CAD build for the part. Positions are in the model's coordinates, mm. A direction names the side the tool comes from. Coordinates: 2 decimals unless noted, no trailing zeros. Loops run counter-clockwise (first coordinate to the right, second up) from the corner with the lowest first, then second, coordinate; pieces in that order, holes last. Notation, with made-up numbers: (-35.5, 48) -> (-21.5, 48) arc R17 cw to (-21.5, 79) -> close; hole circle Ø8 at (-20.75, 21). An arc over 180 degrees is marked (long way). Write each question's results on one line, items separated by ' | '.
```python
from build123d import *

# Parameters (mm, degrees)
SKETCH1_W           = 51.2
SKETCH1_H           = 37.6
BOSS_EXTRUDE1_DEPTH = 2
SKETCH2_W           = 2
SKETCH2_H           = 37.6
BOSS_EXTRUDE2_DEPTH = 37.6
SKETCH3_R           = 1.65
CUT_EXTRUDE2_DEPTH  = 37.6
SKETCH5_R           = 6.6
CUT_EXTRUDE3_DEPTH  = 37.6
SKETCH6_R           = 1.6
CUT_EXTRUDE4_DEPTH  = 37.6
FILLET1_R           = 2
FILLET2_R           = 2
FILLET3_R           = 18.8


with BuildPart() as part:
    # Sketch1 → Boss-Extrude1 (new body)
    with BuildSketch(Plane(origin=(0, 0, 0), x_dir=(1, 0, 0), z_dir=(0, 1, 0))):
        Rectangle(SKETCH1_W, SKETCH1_H)
    extrude(amount=BOSS_EXTRUDE1_DEPTH)

    # Sketch2 → Boss-Extrude2 (add)
    with BuildSketch(Plane(origin=(0, 2, 0), x_dir=(1, 0, 0), z_dir=(0, 1, 0))):
        with Locations((-24.6, 0)):
            Rectangle(SKETCH2_W, SKETCH2_H)
    extrude(amount=BOSS_EXTRUDE2_DEPTH)

    # Sketch3 → Cut-Extrude2 (cut)
    with BuildSketch(Plane.ZY.offset(25.6)):
        with Locations((15.5, 20.8)):
            Circle(SKETCH3_R)
        with Locations((6.883974596, 7.876606241)):
            Circle(SKETCH3_R)
        with Locations((-8.616025404, 8.876606241)):
            Circle(SKETCH3_R)
        with Locations((-15.5, 22.8)):
            Circle(SKETCH3_R)
        with Locations((-6.883974596, 35.723393759)):
            Circle(SKETCH3_R)
        with Locations((8.616025404, 34.723393759)):
            Circle(SKETCH3_R)
    extrude(amount=-CUT_EXTRUDE2_DEPTH, mode=Mode.SUBTRACT)

    # Sketch5 → Cut-Extrude3 (cut)
    with BuildSketch(Plane.ZY.offset(25.6)):
        with Locations((0, 27.8)):
            Circle(SKETCH5_R)
        with BuildLine():
            Line((6.6, 13.8), (6.6, 27.8))
            ThreePointArc((6.6, 27.8), (0, 21.2), (-6.6, 27.8))
            Line((-6.6, 27.8), (-6.6, 13.8))
            ThreePointArc((-6.6, 13.8), (0, 20.4), (6.6, 13.8))
        make_face()
        with Locations((0, 13.8)):
            Circle(SKETCH5_R)
    extrude(amount=-CUT_EXTRUDE3_DEPTH, mode=Mode.SUBTRACT)

    # Sketch6 → Cut-Extrude4 (cut)
    with BuildSketch(Plane(origin=(0, 0, 0), x_dir=(-1, 0, 0), z_dir=(0, -1, 0))):
        with Locations(Location((17.2, -15.6, 0), (0, 0, 90))):
            Circle(SKETCH6_R)
        with Locations(Location((10.8, -15.6, 0), (0, 0, 90))):
            Circle(SKETCH6_R)
        with Locations(Location((4.4, -15.6, 0), (0, 0, 90))):
            Circle(SKETCH6_R)
        with Locations(Location((-2, -15.6, 0), (0, 0, 90))):
            Circle(SKETCH6_R)
        with Locations(Location((-8.4, -15.6, 0), (0, 0, 90))):
            Circle(SKETCH6_R)
        with Locations(Location((-14.8, -15.6, 0), (0, 0, 90))):
            Circle(SKETCH6_R)
        with Locations(Location((-21.2, -15.6, 0), (0, 0, 90))):
            Circle(SKETCH6_R)
        with Locations(Location((-21.2, 15.6, 0), (0, 0, 270))):
            Circle(SKETCH6_R)
        with Locations(Location((-14.8, 15.6, 0), (0, 0, 270))):
            Circle(SKETCH6_R)
        with Locations(Location((-8.4, 15.6, 0), (0, 0, 270))):
            Circle(SKETCH6_R)
        with Locations(Location((-2, 15.6, 0), (0, 0, 270))):
            Circle(SKETCH6_R)
        with Locations(Location((4.4, 15.6, 0), (0, 0, 270))):
            Circle(SKETCH6_R)
        with Locations(Location((10.8, 15.6, 0), (0, 0, 270))):
            Circle(SKETCH6_R)
        with Locations(Location((17.2, 15.6, 0), (0, 0, 270))):
            Circle(SKETCH6_R)
    extrude(amount=-CUT_EXTRUDE4_DEPTH, mode=Mode.SUBTRACT)

    # Fillet1
    fillet1_edges = [part.edges().sort_by_distance(p)[0] for p in [
        (25.6, 1, -18.8),
        (25.6, 1, 18.8),
    ]]
    fillet(fillet1_edges, radius=FILLET1_R)

    # Fillet2
    fillet2_edges = [part.edges().sort_by_distance(p)[0] for p in [
        (-25.6, 0, 0),
    ]]
    fillet(fillet2_edges, radius=FILLET2_R)

    # Fillet3
    fillet3_edges = [part.edges().sort_by_distance(p)[0] for p in [
        (-24.6, 39.6, -18.8),
        (-24.6, 39.6, 18.8),
    ]]
    fillet(fillet3_edges, radius=FILLET3_R - 0.0001)  # a hair under: the kernel refuses the full size


solid = part.part
```
Q1. Which spindle directions (+Z, -Z, +X, -X, +Y, -Y) get a long thin tool onto all of the face, cutting with end or side? Do faces 4 (the cylindrical face through (2.61, 0.99, -14.12)), 5 (the flat face through (-23.6, 21, -8)), 6 (the cylindrical face through (-24.6, 7.2, -0.1)). Say none if no direction does.
Results are:
face 4: +Y, -Y | face 5: +Z, -Z, +X, +Y | face 6: +X, -X
Q2. Drop flat-ended pins along their axis: pin 1 (5 mm diameter, centred on x = 21.2, z = -15.6, fed in from +Y); pin 2 (4.5 mm diameter, centred on y = 8.88, z = -8.62, fed in from +X). Give the stop position or say it passes through.
Results are:
pin 1: y = 2 | pin 2: x = -23.6
Q3. Wall check: L1, parallel to Z at x = -24, y = 20; L2, parallel to X at y = 6, z = -17; L3, parallel to Y at x = 19, z = 16. Give the ranges that are in metal, low to high. Write a range as from..to.
Results are:
L1: -18.8..-6.6, 6.6..14.06, 16.94..18.8 | L2: -25.6..-23.6 | L3: 0..2
Q4. Cut at C-C on z = -3. Write the cut outline in (x, y), and give its area (3 significant figures).
Results are:
outline: (-25.6, 2) arc R2 ccw to (-23.6, 0) -> (25.6, 0) -> (25.6, 2) -> (-23.6, 2) -> (-23.6, 7.92) -> (-25.6, 7.92) -> close; (-25.6, 33.68) -> (-23.6, 33.68) -> (-23.6, 39.36) -> (-25.6, 39.36) -> close | area: 125 mm^2
Q5. Cut at A-A on x = -17.2. Write the cut outline in (y, z).
Results are:
outline: (0, -18.8) -> (2, -18.8) -> (2, -17.2) -> (0, -17.2) -> close; (0, -14) -> (2, -14) -> (2, 14) -> (0, 14) -> close; (0, 17.2) -> (2, 17.2) -> (2, 18.8) -> (0, 18.8) -> close
Q6. Cut at D-D on x = -5. Write the cut outline in (y, z).
Results are:
outline: (0, -18.8) -> (2, -18.8) -> (2, -17.08) -> (0, -17.08) -> close; (0, -14.12) -> (2, -14.12) -> (2, 14.12) -> (0, 14.12) -> close; (0, 17.08) -> (2, 17.08) -> (2, 18.8) -> (0, 18.8) -> close
Q7. Pull direction Z, two halves, no side cores. Call faces 1 (the cylindrical face through (-16.59, 0.99, -14.12)), 2 (the flat face through (-7, 1, 18.8)), 3 (the flat face through (1, 2, 0)): +Z half, -Z half, draft (parallel to the pull), parting line (faces both ways), or undercut.
Results are:
face 1: undercut | face 2: +Z half | face 3: draft
Q8. Cut at B-B on y = 18.5. Write the cut outline in (x, z), and give its area (3 significant figures).
Results are:
outline: (-25.6, -18.8) -> (-23.6, -18.8) -> (-23.6, -6.6) -> (-25.6, -6.6) -> close; (-25.6, 6.6) -> (-23.6, 6.6) -> (-23.6, 18.8) -> (-25.6, 18.8) -> close | area: 48.8 mm^2
